Check sheet for the drawn part. Datum: minimum x, y, z corner. Units: mm. A direction names the side the tool comes from. Give positions to 0.01 mm unless a question says otherwise; leave off trailing zeros. Order: outer loops, then holes, each group sorted by start corner. A loop starts at its lowest first (then second) coordinate and runs counter-clockwise, first axis right, second up. Notation, with made-up numbers: (84.25, -20) - (116.25, -20) arc R29 ccw to (116.25, 5) - close; hole circle Ø5 at (-2, 37.5). An arc over 180 degrees is marked (long way). Answer as a JSON object with one key per item and string values. Group by question number.
(1) Mould release check, pull along Y, two halves, no side actions. Record for the marked faces 3, 4 and 5: +Y half, -Y half, draft (parallel to the pull), parting line (faces both ways), or undercut.
(2) Section check C-C (y = 5.5). Record the boundary of the cut face in (x, z), then the cut area to 3 significant figures.
(3) Thickness scan on line 1 (X direction, y = 4.5, z = 0.2). Record the ranges inside material, lowest first.
(4) Depth check by flat-ended pin: pin 1 Ø0.8 at (x, z) = (0.5, 1) entering from +Y; pin 2 Ø1.2 at (x, z) = (5, 2.5) entering from +Y; pin 3 Ø0.6 at (y, z) = (5, 1) entering from +X. Enter the tip coordinate at first touch or a pass-through.
(5) Section check B-B (x = 1.2). Record the boundary of the cut face in (y, z).
(6) Access from +Z, -Z, +X, -X, +Y, -Y to the whole of each face (thin tool, end or side, straight path). Record for the marked faces 1 and 2.
(7) Section check A-A (z = 0.75). Record the boundary of the cut face in (x, y).
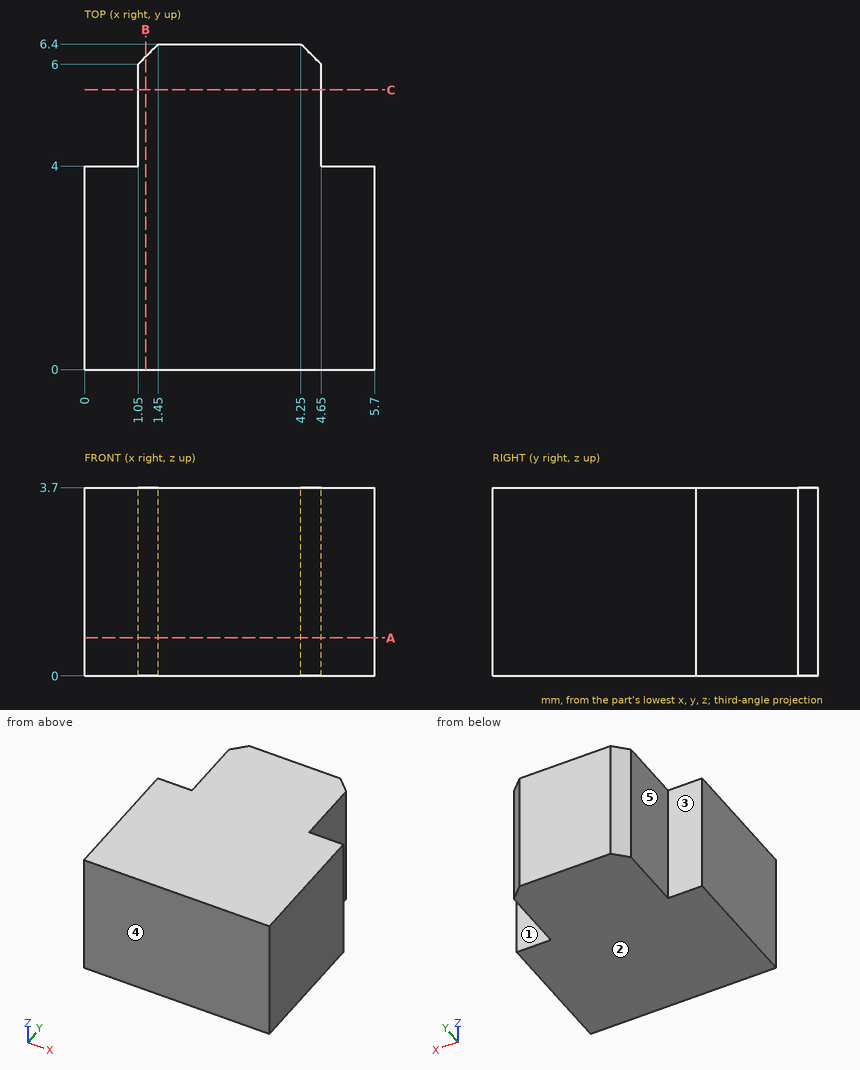
Solutions:
{
 "1": {"face 3": "+Y half", "face 4": "-Y half", "face 5": "draft"},
 "2": {"outline": "(1.05, 0) - (4.65, 0) - (4.65, 3.7) - (1.05, 3.7) - close", "area": "13.3 mm2"},
 "3": {"line 1": "x = 1.05 to 4.65"},
 "4": {"pin 1": "stops at y = 4", "pin 2": "stops at y = 6.25", "pin 3": "stops at x = 4.65"},
 "5": {"outline": "(0, 0) - (6.15, 0) - (6.15, 3.7) - (0, 3.7) - close"},
 "6": {"face 1": "+Z, -Z, +X, +Y", "face 2": "-Z, +X, -X, +Y, -Y"},
 "7": {"outline": "(0, 0) - (5.7, 0) - (5.7, 4) - (4.65, 4) - (4.65, 6) - (4.25, 6.4) - (1.45, 6.4) - (1.05, 6) - (1.05, 4) - (0, 4) - close"}
}
